from build123d import *

# Parameters (mm, degrees)
BOSS_EXTRUDE1_DEPTH     = 20.95
BOSS_EXTRUDE2_START     = -9.05
BOSS_EXTRUDE2_DEPTH     = 9.05
SKETCH6_R               = 2.2
CUT_EXTRUDE2_DEPTH      = 10
CUT_EXTRUDE3_DEPTH      = 2.75
CUT_EXTRUDE4_DEPTH      = 67.499081444
CUT_EXTRUDE4_DEPTH_BACK = 67.499081444
SKETCH8_W               = 8.290514233
SKETCH8_H               = 3.25
SKETCH11_R              = 11.25
BEARING_HOLE_DEPTH      = 7.6
SKETCH9_W               = 12.3
SKETCH9_H               = 21.5
WIRE_HOLE_DEPTH         = 62.274898109
SKETCH12_W              = 46
SKETCH12_H              = 30
BOSS_EXTRUDE3_DEPTH     = 0.0001
BOSS_EXTRUDE4_DEPTH     = 7.5
BOSS_EXTRUDE5_START     = -7.5
BOSS_EXTRUDE5_DEPTH     = 7.5
BOSS_EXTRUDE9_START     = 2.5
BOSS_EXTRUDE9_DEPTH     = 2.5
SKETCH15_R              = 4
CUT_EXTRUDE5_DEPTH      = 77.054456365
SKETCH17_R              = 6.169612062
SHAT_HOLE_DEPTH         = 10
SKETCH18_R              = 4
BOSS_EXTRUDE7_DEPTH     = 14
SKETCH19_R              = 4.675
CUT_EXTRUDE6_DEPTH      = 2
SKETCH24_R              = 5
CUT_EXTRUDE7_DEPTH      = 65.382744838
FILLET1_R               = 1
SKETCH25_W              = 8.843315878
SKETCH25_H              = 4.834346013
BOSS_EXTRUDE10_DEPTH    = 2
SKETCH27_W              = 12.3
SKETCH27_H              = 21.5
CUT_EXTRUDE8_DEPTH      = 60.56786481
BOSS_EXTRUDE11_DEPTH    = 14.5901
CUT_EXTRUDE9_REACH      = 69.405
SKETCH29_W              = 15.2
SKETCH29_H              = 3
CUT_EXTRUDE14_START     = -10.25
CUT_EXTRUDE14_DEPTH     = 10.25
SKETCH34_R              = 6.901355235
CUT_EXTRUDE15_DEPTH     = 5
FILLET2_R               = 0.5
SKETCH35_R              = 2.2
CUT_EXTRUDE16_DEPTH     = 6.7
CUT_EXTRUDE17_DEPTH     = 10.25
CUT_EXTRUDE18_REACH     = 69.405


with BuildPart() as part:
    # Sketch2 → Boss-Extrude1 (new body)
    with BuildSketch(Plane.XY):
        with BuildLine():
            Line((-14.709485767, 40), (-23, 40))
            Line((-23, 40), (-23, 0))
            Line((-23, 0), (23, 0))
            Line((23, 0), (23, 40))
            Line((23, 40), (14.709485767, 40))
            ThreePointArc((14.709485767, 40), (0, 54.709485767), (-14.709485767, 40))
        make_face()
        with BuildLine():
            Line((-7.65, 18.18111404), (-7.65, 14.59))
            Line((-7.65, 14.59), (7.65, 14.59))
            Line((7.65, 14.59), (7.65, 18.18111404))
            Line((7.65, 18.18111404), (9.45, 18.18111404))
            Line((9.45, 18.18111404), (9.45, 21.20025831))
            ThreePointArc((9.45, 21.20025831), (0, 46.349332344), (-9.45, 21.20025831))
            Line((-9.45, 21.20025831), (-9.45, 18.18111404))
            Line((-9.45, 18.18111404), (-7.65, 18.18111404))
        make_face(mode=Mode.SUBTRACT)
    extrude(amount=BOSS_EXTRUDE1_DEPTH)

    # Sketch3 → Boss-Extrude2 (add)
    with BuildSketch(Plane.XY.offset(BOSS_EXTRUDE2_START)):
        with BuildLine():
            Line((-14.709485767, 40), (-23, 40))
            Line((-23, 40), (-23, 0))
            Line((-23, 0), (23, 0))
            Line((23, 0), (23, 40))
            Line((23, 40), (14.709485767, 40))
            ThreePointArc((14.709485767, 40), (0, 54.709485767), (-14.709485767, 40))
        make_face()
    extrude(amount=BOSS_EXTRUDE2_DEPTH)

    # Sketch6 → Cut-Extrude2 (cut)
    with BuildSketch(Plane.XY.offset(20.95)):
        with Locations((-17.5, 32)):
            Circle(SKETCH6_R)
        with Locations((17.5, 32)):
            Circle(SKETCH6_R)
    extrude(amount=-CUT_EXTRUDE2_DEPTH, mode=Mode.SUBTRACT)

    # Sketch7 → Cut-Extrude3 (cut)
    with BuildSketch(Plane.XY.offset(20.95)):
        with BuildLine():
            Line((-17.7, 35.75), (17.3, 35.75))
            ThreePointArc((17.3, 35.75), (21.05, 32), (17.3, 28.25))
            Line((17.3, 28.25), (-17.7, 28.25))
            ThreePointArc((-17.7, 28.25), (-21.45, 32), (-17.7, 35.75))
        make_face()
    extrude(amount=-CUT_EXTRUDE3_DEPTH, mode=Mode.SUBTRACT)

    # Sketch8 → Cut-Extrude4 (cut, two sides: drawn at the far end of the back side and taken through both)
    with BuildSketch(Plane.XY.offset(20.95).offset(-CUT_EXTRUDE4_DEPTH_BACK)):
        with Locations((-18.854742884, 38.375)):
            Rectangle(SKETCH8_W, SKETCH8_H)
        with Locations((18.854742884, 38.375)):
            Rectangle(SKETCH8_W, SKETCH8_H)
    extrude(amount=CUT_EXTRUDE4_DEPTH + CUT_EXTRUDE4_DEPTH_BACK, mode=Mode.SUBTRACT)

    # Sketch11 → Bearing Hole (cut)
    with BuildSketch(Plane(origin=(0, 0, -9.05), x_dir=(-1, 0, 0), z_dir=(0, 0, -1))):
        with Locations((0, 40)):
            Circle(SKETCH11_R)
    extrude(amount=-BEARING_HOLE_DEPTH, mode=Mode.SUBTRACT)

    # Sketch9 → Wire Hole (cut, through all)
    with BuildSketch(Plane(origin=(0, 14.59, -19.25), x_dir=(-1, 0, 0), z_dir=(0, 1, 0))):
        with Locations((0, 26.95)):
            Rectangle(SKETCH9_W, SKETCH9_H)
    extrude(amount=-WIRE_HOLE_DEPTH, mode=Mode.SUBTRACT)

    # Sketch12 → Boss-Extrude3 (add)
    with BuildSketch(Plane.XZ):
        with Locations((0, 5.95)):
            Rectangle(SKETCH12_W, SKETCH12_H)
    extrude(amount=BOSS_EXTRUDE3_DEPTH)

    # Sketch13 → Boss-Extrude4 (add)
    with BuildSketch(Plane(origin=(23, 0, 0), x_dir=(0, 0, -1), z_dir=(1, 0, 0))):
        with BuildLine():
            Line((-20.95, -0.0001), (-20.95, -20.0001))
            ThreePointArc((-20.95, -20.0001), (-5.95, -35.0001), (9.05, -20.0001))
            Line((9.05, -20.0001), (9.05, -0.0001))
            Line((9.05, -0.0001), (-20.95, -0.0001))
        make_face()
    extrude(amount=-BOSS_EXTRUDE4_DEPTH)

    # Sketch14 → Boss-Extrude5 (add)
    with BuildSketch(Plane.ZY.offset(23).offset(BOSS_EXTRUDE5_START)):
        with BuildLine():
            Line((-9.05, -20.0001), (-9.05, -0.0001))
            Line((-9.05, -0.0001), (20.95, -0.0001))
            Line((20.95, -0.0001), (20.95, -20.0001))
            ThreePointArc((20.95, -20.0001), (5.95, -35.0001), (-9.05, -20.0001))
        make_face()
    extrude(amount=BOSS_EXTRUDE5_DEPTH)

    # Sketch21 → Boss-Extrude9 (add)
    with BuildSketch(Plane(origin=(23, 0, 0), x_dir=(0, 0, -1), z_dir=(1, 0, 0)).offset(BOSS_EXTRUDE9_START)):
        with BuildLine():
            Line((-20.95, -20.0001), (-20.95, 36.75))
            Line((-20.95, 36.75), (9.05, 36.75))
            Line((9.05, 36.75), (9.05, -20.0001))
            ThreePointArc((9.05, -20.0001), (-5.95, -35.0001), (-20.95, -20.0001))
        make_face()
    extrude(amount=-BOSS_EXTRUDE9_DEPTH)

    # Sketch15 → Cut-Extrude5 (cut, through all)
    with BuildSketch(Plane.ZY.offset(23)):
        with Locations(Location((5.95, -20.0001, 0), (0, 0, 270))):
            Circle(SKETCH15_R)
    extrude(amount=-CUT_EXTRUDE5_DEPTH, mode=Mode.SUBTRACT)

    # Sketch17 → Shat hole (add)
    with BuildSketch(Plane(origin=(25.5, 0, -23), x_dir=(0, 0, 1), z_dir=(-1, 0, 0))):
        with Locations((28.95, -20.0001)):
            Circle(SKETCH17_R)
        with BuildLine():
            Line((26.876355865, -18.3501), (31.023644135, -18.3501))
            ThreePointArc((31.023644135, -18.3501), (31.6, -20.0001), (31.023644135, -21.6501))
            Line((31.023644135, -21.6501), (26.876355865, -21.6501))
            ThreePointArc((26.876355865, -21.6501), (26.3, -20.0001), (26.876355865, -18.3501))
        make_face(mode=Mode.SUBTRACT)
    extrude(amount=SHAT_HOLE_DEPTH)

    # Sketch18 → Boss-Extrude7 (add)
    with BuildSketch(Plane.ZY.offset(23)):
        with Locations(Location((5.95, -20.0001, 0), (0, 0, 270))):
            Circle(SKETCH18_R)
    extrude(amount=-BOSS_EXTRUDE7_DEPTH)

    # Sketch19 → Cut-Extrude6 (cut)
    with BuildSketch(Plane.ZY.offset(-15.5)):
        with Locations((5.95, -20.0001)):
            Circle(SKETCH19_R)
    extrude(amount=-CUT_EXTRUDE6_DEPTH, mode=Mode.SUBTRACT)

    # Sketch24 → Cut-Extrude7 (cut, through all)
    with BuildSketch(Plane(origin=(0, 0, -1.45), x_dir=(-1, 0, 0), z_dir=(0, 0, -1))):
        with Locations((0, 40)):
            Circle(SKETCH24_R)
    extrude(amount=-CUT_EXTRUDE7_DEPTH, mode=Mode.SUBTRACT)

    # Fillet1
    fillet1_edges = [part.edges().sort_by_distance(p)[0] for p in [
        (11.25, 40, -9.05),
    ]]
    fillet(fillet1_edges, radius=FILLET1_R)

    # Sketch25 → Boss-Extrude10 (add)
    with BuildSketch(Plane(origin=(25.5, 0, 0), x_dir=(0, 0, -1), z_dir=(1, 0, 0))):
        with Locations((-6.185865257, -20.38943492)):
            Rectangle(SKETCH25_W, SKETCH25_H)
    extrude(amount=-BOSS_EXTRUDE10_DEPTH)

    # Sketch27 → Cut-Extrude8 (cut, through all)
    with BuildSketch(Plane(origin=(0, 14.59, 0), x_dir=(1, 0, 0), z_dir=(0, 1, 0))):
        with Locations((0, -7.7)):
            Rectangle(SKETCH27_W, SKETCH27_H)
    extrude(amount=-CUT_EXTRUDE8_DEPTH, mode=Mode.SUBTRACT)

    # Sketch28 → Boss-Extrude11 (add)
    with BuildSketch(Plane.XZ.offset(0.0001)):
        Polygon((-6.15, 7.7), (0, 17.95), (6.15, 7.7), (6.15, 18.45), (-6.15, 18.45), align=None)
    extrude(amount=-BOSS_EXTRUDE11_DEPTH)

    # Cut-Extrude9: up to this face of the body (flat: up to its plane)
    cut_extrude9_end = Plane(part.part.faces().sort_by_distance((0, 29.436315862, 0))[0])
    # Sketch29 → Cut-Extrude9 (cut, up to the picked face)
    with BuildSketch(Plane.XY.offset(20.95), mode=Mode.PRIVATE) as cut_extrude9_sk1:
        with Locations((-0.05, 13.09)):
            Rectangle(SKETCH29_W, SKETCH29_H)
    cut_extrude9_tool1 = split(extrude(cut_extrude9_sk1.sketch, amount=-CUT_EXTRUDE9_REACH, mode=Mode.PRIVATE), bisect_by=cut_extrude9_end, keep=Keep.BOTH, mode=Mode.PRIVATE)
    add(cut_extrude9_tool1.solids().sort_by(Axis((-0.05, 13.09, 20.95), (0, 0, -1)))[0], mode=Mode.SUBTRACT)

    # Sketch33 → Cut-Extrude14 (cut)
    with BuildSketch(Plane.ZY.offset(23).offset(CUT_EXTRUDE14_START)):
        with BuildLine():
            Line((-4.35, 11.89), (16.25, 11.89))
            Line((16.25, 11.89), (11.25, 0.2999))
            Line((11.25, 0.2999), (20.95, 0.2999))
            Line((20.95, 0.2999), (20.95, -20.0001))
            ThreePointArc((20.95, -20.0001), (5.95, -35.0001), (-9.05, -20.0001))
            Line((-9.05, -20.0001), (-9.05, 0.2999))
            Line((-9.05, 0.2999), (0.65, 0.2999))
            Line((0.65, 0.2999), (-4.35, 11.89))
        make_face()
    extrude(amount=CUT_EXTRUDE14_DEPTH, mode=Mode.SUBTRACT)


with BuildPart() as cut_extrude14_piece_1:
    # of the separate pieces the step leaves, piece 1, a body of its own (cut_extrude14_pieces)
    add(part.part.solids().sort_by_distance((14.709485767, 40, -9.05))[0])

    # Fillet2
    fillet2_edges = [cut_extrude14_piece_1.edges().sort_by_distance(p)[0] for p in [
        (-17.875, 0.2999, 11.25),
        (-17.875, 0.2999, 0.65),
    ]]
    fillet(fillet2_edges, radius=FILLET2_R)

    # Sketch35 → Cut-Extrude16 (cut)
    with BuildSketch(Plane.ZY.offset(12.75)):
        with Locations(Location((5.95, 5.89, 0), (0, 0, 270))):
            Circle(SKETCH35_R)
    extrude(amount=-CUT_EXTRUDE16_DEPTH, mode=Mode.SUBTRACT)

    # Sketch36 → Cut-Extrude17 (cut)
    with BuildSketch(Plane.ZY.offset(23)):
        with BuildLine():
            Line((-3.953885576, 10.971798844), (-4.35, 11.89))
            Line((-4.35, 11.89), (-3.35, 11.89))
            ThreePointArc((-3.35, 11.89), (-5.185498182, 12.43949321), (-3.953885576, 10.971798844))
        make_face()
        with BuildLine():
            Line((15.853885576, 10.971798844), (16.25, 11.89))
            Line((16.25, 11.89), (15.25, 11.89))
            ThreePointArc((15.25, 11.89), (17.085498182, 12.43949321), (15.853885576, 10.971798844))
        make_face()
    extrude(amount=-CUT_EXTRUDE17_DEPTH, mode=Mode.SUBTRACT)

    # Sketch37 → Cut-Extrude18 (cut, up to next)
    with BuildSketch(Plane.XY.offset(20.95), mode=Mode.PRIVATE) as cut_extrude18_sk1:
        Polygon((6.15, -0.0001), (6.15, 7.9999), (-1.95, 7.9999), (-1.95, 2.9999), (4.4, 2.9999), (4.4, -0.0001), align=None)
    cut_extrude18_tool1 = extrude(cut_extrude18_sk1.sketch, amount=-CUT_EXTRUDE18_REACH, mode=Mode.PRIVATE) & cut_extrude14_piece_1.part
    add(cut_extrude18_tool1.solids().sort_by_distance((2.464344, 5.040884, 20.95))[0], mode=Mode.SUBTRACT)


with BuildPart() as cut_extrude14_piece_2:
    # of the separate pieces the step leaves, piece 2, a body of its own (cut_extrude14_pieces)
    add(part.part.solids().sort_by_distance((-12.75, -24.0001, 5.95))[0])

    # Sketch34 → Cut-Extrude15 (cut)
    with BuildSketch(Plane.ZY.offset(12.75)):
        with Locations((5.95, -20.0001)):
            Circle(SKETCH34_R)
    extrude(amount=-CUT_EXTRUDE15_DEPTH, mode=Mode.SUBTRACT)


solid = cut_extrude14_piece_1.part
Read the model definition and answer for the solid it produces. Units are mm, in the model's axes. A direction names the side the tool comes from. Give positions to 0.01 mm unless a question says otherwise; leave off trailing zeros. Write each loop counter-clockwise with the first axis right and the second up, starting at its lowest first coordinate (ties: lowest second). Pieces come first, ordered by that corner, then holes. Notation, with made-up numbers: (63.25, 25.25) - (71.25, 25.25) arc R24 ccw to (71.25, 42.25) - close; hole circle Ø10 at (-5.75, 69). An arc over 180 degrees is marked (long way). Answer in a Markdown table with one row per item. Add a question column.
Item 1: Determine the mould class of faces 5 (the face through (0.49, 46.34, 10.33)), 6 (the face through (-18, 11.89, 6)), 7 (the face through (1.465, 51.154, -4.796)), 8 (the face through (-12.75, 9, 6)) for opening direction X: pulls with the +X half, pulls with the -X half, needs draft (parallel to the pull), parting line crosses it, or undercut.
Item 2: Find the intervals of material crossed by L1, parallel to Y at x = 16, z = 5.95; L2, parallel to Y at x = 0, z = -4; L3, parallel to X at y = 3.5, z = -0.5, in increasing order.
Item 3: Section B-B, the plane y = -10 is taken. Write down the section's boundary in (x, z).
Item 4: A tool of negligible diameter and unlimited length cuts with its end or side. For faces 1 (the face through (-5, 38, -1.45)), 2 (the face through (20, 36.75, 6)), 3 (the face through (-16.48, 30.05, 14.63)), 4 (the face through (17.5, -22, 6)), from which of +Z, -Z, +X, -X, +Y, -Y can it reach the whole face along a straight path? Write none if from no direction.
Item 5: Section A-A, the plane y = 19.5 is taken. Write down the section's boundary in (x, z), and give its area (3 significant figures).
Item 6: Flat-ended cylindrical pins translate along their axes: P1, Ø8, axis at x = 19, y = 37, coming from the +Z side; P2, Ø1, axis at y = -20.5, z = 7, coming from the -X side; P3, Ø8, axis at x = 13, z = 13, coming from the +Y side; P4, Ø3, axis at x = 15, z = 20, coming from the -Y side. Find the tip coordinate at first contact, or state that the pin passes through.
Item 7: Section C-C, the plane y = -23.5 is taken. Write down the section's boundary in (x, z), and give its area (3 significant figures).
Recorded:
| question | item | result |
|---|---|---|
| 1 | face 5 | undercut |
| 1 | face 6 | needs draft |
| 1 | face 7 | undercut |
| 1 | face 8 | pulls with the -X half |
| 2 | L1 | y = -35 to -24.68, -15.33 to 36.75 |
| 2 | L2 | y = 0 to 28.75, 51.25 to 54.71 |
| 2 | L3 | x = -12.75 to -6.15, 6.15 to 25.5 |
| 3 | outline | (15.5, -9.05) - (25.5, -9.05) - (25.5, 20.95) - (15.5, 20.95) - close |
| 4 | face 1 | -Z |
| 4 | face 2 | +Z, -Z, +X, +Y |
| 4 | face 3 | +Z |
| 4 | face 4 | -X |
| 5 | outline | (-23, -9.05) - (25.5, -9.05) - (25.5, 20.95) - (9.45, 20.95) - (9.45, 0) - (-9.45, 0) - (-9.45, 20.95) - (-23, 20.95) - close |
| 5 | area | 1,060 mm2 |
| 6 | P1 | stops at z = 20.95 |
| 6 | P2 | stops at x = 23.5 |
| 6 | P3 | stops at y = 51.63 |
| 6 | P4 | stops at y = -28.08 |
| 7 | outline | (15.5, -8.64) - (25.5, -8.64) - (25.5, 20.54) - (15.5, 20.54) - (15.5, 9.05) - (17.5, 9.05) - (17.5, 2.85) - (15.5, 2.85) - close |
| 7 | area | 279 mm2 |
